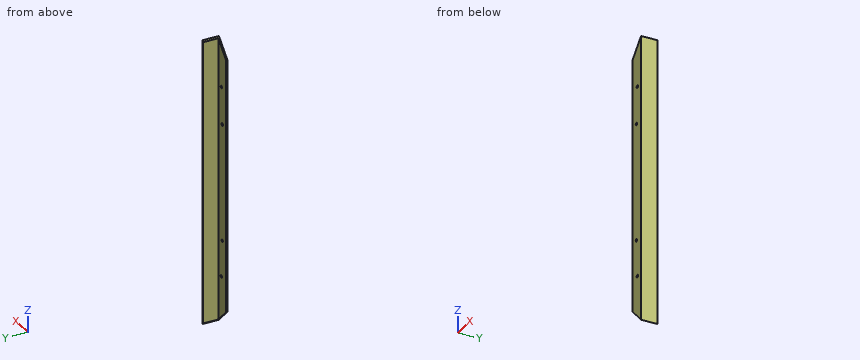
Autodesk Inventor part; units mm, degrees
ref_plane "YZ Plane" through (0, 0, 0) normal (1, 0, 0) x (0, 1, 0)
ref_plane "XZ Plane" through (0, 0, 0) normal (0, 1, 0) x (-1, 0, 0)
ref_plane "XY Plane" through (0, 0, 0) normal (0, 0, 1) x (1, 0, 0)
sketch "Sketch1" plane through (0, 0, 0) normal (0, 1, 0) x (-1, 0, 0)
  line L0 (0, 0) -> (0, -650)
  line L1 (0, -650) -> (650, -650)
  line L2 (650, -650) -> (650, 0)
  line L3 (650, 0) -> (0, 0)
  line L4 (0, 0) -> (3, 0)
  line L5 (3, -3) -> (3, -647)
  line L6 (3, -650) -> (0, -650)
  line L7 (0, -650) -> (0, -647)
  line L8 (650, -647) -> (650, -650)
  line L9 (650, -650) -> (647, -650)
  line L10 (647, -650) -> (647, 0)
  line L11 (647, 0) -> (650, 0)
  line L12 (650, 0) -> (650, -3)
  line L13 (0, -3) -> (0, 0)
  line L14 (0, 0) -> (0, -37)
  line L15 (650, -37) -> (650, 0)
  line L16 (650, 0) -> (613, 0)
  line L17 (613, 0) -> (613, -650)
  line L18 (613, -650) -> (650, -650)
  line L19 (650, -650) -> (650, -613)
  line L20 (0, -613) -> (0, -650)
  line L21 (0, -650) -> (37, -650)
  line L22 (37, 0) -> (0, 0)
  line L23 (3, -147.3087) -> (3, -94.9828)
  line L24 (147.3087, -3) -> (94.9828, -3)
  circle A0 centre (16.1109, -108.0348) radius 3
  line L25 (0, -650) -> (3, -650)
  line L26 (0, -647) -> (0, -650)
  line L27 (0, -650) -> (0, -613)
  line L28 (37, -650) -> (0, -650)
  line L29 (3, -502.6913) -> (3, -555.0172)
  line L30 (147.3087, -647) -> (94.9828, -647)
  circle A1 centre (16.1109, -541.9652) radius 3
  line L31 (37, -650) -> (37, -37)
  line L32 (37, -3) -> (37, 0)
  line L33 (650, -3) -> (34.9546, -3)
  line L34 (34.9546, -647) -> (650, -647)
  line L35 (37, -37) -> (0, 0)
  line L36 (37, -613) -> (0, -650)
  line L37 (0, -650) -> (3, -647)
  line L38 (3, -647) -> (3, -3)
  line L39 (3, -3) -> (0, 0)
  line L40 (3, -325) -> (3, -458)
  line L41 (3, -458) -> (20, -458)
  line L42 (3, -325) -> (3, -192)
  line L43 (3, -192) -> (20, -192)
  circle A2 centre (20, -192) radius 3
  circle A3 centre (20, -458) radius 3
  line L44 (325, -650) -> (192, -650)
  line L45 (192, -650) -> (192, -630)
  circle A4 centre (192, -630) radius 3
  line L46 (3, -458) -> (3, -475)
  line L47 (3, -475) -> (647, -475)
  line L48 (3, -475) -> (3, -478)
  line L49 (3, -478) -> (647, -478)
  line L50 (192, -630) -> (175, -630)
  line L51 (192, -630) -> (209, -630)
  line L52 (209, -630) -> (209, -478)
  line L53 (175, -630) -> (175, -478)
  point P0 (37, -647)
  dimension "d0" = 650
  dimension "d1" = 650
  dimension "d2" = 650
  dimension "d3" = 3
  dimension "d4" = 650
  dimension "d5" = 3
  dimension "d6" = 3
  dimension "d7" = 650
  dimension "d8" = 3
  dimension "d9" = 650
  dimension "d10" = 37
  dimension "d12" = 37
  dimension "d13" = 650
  dimension "d14" = 37
  dimension "d15" = 650
  dimension "d16" = 37
  dimension "d28" = 6
  dimension "d33" = 133
  dimension "d34" = 17
  dimension "d35" = 133
  dimension "d36" = 17
  dimension "d37" = 6
  dimension "d38" = 6
  dimension "d41" = 133
  dimension "d42" = 20
  dimension "d43" = 6
  dimension "d44" = 17
  dimension "d45" = 3
  dimension "d46" = 17
  dimension "d47" = 17
extrude "Extrusion1" add sketch "Sketch1" along normal blind 3 contours L35 L5 L36 L0 | A2 | A3 | L35 L31 L47 L5 | L31 L49 L5 L47 | L31 L36 L5 L49
extrude "Extrusion2" add sketch "Sketch1" along normal blind 37 contours L35 L5 L36 L0
extrude "Extrusion3" cut sketch "Sketch1" along normal blind 3 contours A2 | A3
properties part number "body_outer_L"
Work out the finished part from the listing and answer in its coordinate system (mm). Round coordinates to 2 decimals unless told otherwise and drop trailing zeros. Loops run counter-clockwise (first coordinate to the right, second up) from the corner with the lowest first, then second, coordinate; pieces in that order, holes last. Notation, with made-up numbers: M -11.75,-35 L 29.25,-35 A13 ccw 29.25,-27 Z; hole C -8,-21 d7. An arc over 180 degrees is marked long. One line per question, with ' | ' between items.
Q1. Find section B-B, the plane y = 15. Give the vertices of the cut face in (x, z).
Conclusion:
outline: M -3,-647 L 0,-650 L 0,0 L -3,-3 Z
Q2. Find section A-A, the plane z = -467. Give the vertices of the cut face in (x, y), then the cut area to 3 significant figures.
Conclusion:
outline: M -37,0 L 0,0 L 0,37 L -3,37 L -3,3 L -37,3 Z | area: 213 mm2
Q3. Consider line 1 along X through (y, z) = (1, -192); line 2 along Z through (x, y) = (-20, 0.85); line 3 along X through (y, z) = (15, -79). Determine where each line is inside the solid, lowest interval first. Write a range as from..to.
Conclusion:
line 1: x = -37..-23, -17..0 | line 2: z = -630..-461, -455..-195, -189..-20 | line 3: x = -3..0
Q4. Each of these flat-tipped pins is pushed along its axis until it touches: pin 1 Ø12 at (x, z) = (-32.5, -102.5) entering from +Y; pin 2 Ø17 at (y, z) = (17, -167) entering from -X; pin 3 Ø5.5 at (x, z) = (-20, -458) entering from -Y. Where does it stop, or does it pass through?
Conclusion:
pin 1: stops at y = 3 | pin 2: stops at x = -3 | pin 3: passes through
